from build123d import *

# Parameters (mm, degrees)
BOSS_EXTRUDE1_START = -72.4
SKETCH1_W           = 25.6
SKETCH1_H           = 1.2
BOSS_EXTRUDE1_DEPTH = 16.8
BOSS_EXTRUDE2_START = -71.8
SKETCH2_W           = 24.4
SKETCH2_H           = 1.21
BOSS_EXTRUDE2_DEPTH = 15.6
BOSS_EXTRUDE3_START = -72.1
SKETCH3_W           = 1
SKETCH3_H           = 1.1
BOSS_EXTRUDE3_DEPTH = 0.31
BOSS_EXTRUDE4_START = -56.21
SKETCH4_W           = 1
SKETCH4_H           = 1.1
BOSS_EXTRUDE4_DEPTH = 0.31
BOSS_EXTRUDE5_START = -72.1
SKETCH5_W           = 1
SKETCH5_H           = 1.1
BOSS_EXTRUDE5_DEPTH = 0.31
BOSS_EXTRUDE6_START = -56.21
SKETCH6_W           = 1
SKETCH6_H           = 1.1
BOSS_EXTRUDE6_DEPTH = 0.31
BOSS_EXTRUDE7_START = -72.5
SKETCH7_W           = 3
SKETCH7_H           = 0.7
BOSS_EXTRUDE7_DEPTH = 0.9


with BuildPart() as part:
    # Sketch1 → Boss-Extrude1 (new body)
    with BuildSketch(Plane.XY.offset(BOSS_EXTRUDE1_START)):
        with Locations((-26.8, 0.6)):
            Rectangle(SKETCH1_W, SKETCH1_H)
    extrude(amount=BOSS_EXTRUDE1_DEPTH)

    # Sketch2 → Boss-Extrude2 (add)
    with BuildSketch(Plane.XY.offset(BOSS_EXTRUDE2_START)):
        with Locations((-26.8, 1.795)):
            Rectangle(SKETCH2_W, SKETCH2_H)
    extrude(amount=BOSS_EXTRUDE2_DEPTH)

    # Sketch3 → Boss-Extrude3 (add)
    with BuildSketch(Plane.XY.offset(BOSS_EXTRUDE3_START)):
        with Locations((-21.4, 1.85)):
            Rectangle(SKETCH3_W, SKETCH3_H)
    extrude(amount=BOSS_EXTRUDE3_DEPTH)

    # Sketch4 → Boss-Extrude4 (add)
    with BuildSketch(Plane.XY.offset(BOSS_EXTRUDE4_START)):
        with Locations((-21.4, 1.85)):
            Rectangle(SKETCH4_W, SKETCH4_H)
    extrude(amount=BOSS_EXTRUDE4_DEPTH)

    # Sketch5 → Boss-Extrude5 (add)
    with BuildSketch(Plane.XY.offset(BOSS_EXTRUDE5_START)):
        with Locations((-32.2, 1.85)):
            Rectangle(SKETCH5_W, SKETCH5_H)
    extrude(amount=BOSS_EXTRUDE5_DEPTH)

    # Sketch6 → Boss-Extrude6 (add)
    with BuildSketch(Plane.XY.offset(BOSS_EXTRUDE6_START)):
        with Locations((-32.2, 1.85)):
            Rectangle(SKETCH6_W, SKETCH6_H)
    extrude(amount=BOSS_EXTRUDE6_DEPTH)


with BuildPart() as body_2:
    # Sketch7 → Boss-Extrude7 (new body)
    with BuildSketch(Plane.XY.offset(BOSS_EXTRUDE7_START)):
        with Locations((-26.8, 0.25)):
            Rectangle(SKETCH7_W, SKETCH7_H)
    extrude(amount=BOSS_EXTRUDE7_DEPTH)


with BuildPart() as part_1:
    add(part.part)

    # Combine1: cut body 2
    add(body_2.part, mode=Mode.SUBTRACT)


solid = part_1.part
For this review, take the finished solid that the model builds, in its own axes (mm). A direction names the side the tool comes from. Round coordinates to 2 decimals unless told otherwise and drop trailing zeros. Order: outer loops, then holes, each group sorted by start corner. A loop starts at its lowest first (then second) coordinate and runs counter-clockwise, first axis right, second up. Notation, with made-up numbers: M 51.25,-6 L 76.25,-6 A24 cw 76.25,27 Z; hole C -22,0.25 d5. An arc over 180 degrees is marked long. Use a Markdown table: item, result. Add a question column.
Item 1: Tool access review of faces 1 (the flat face through (-39, 2, -64)), 2 (the flat face through (-27, 0.6, -72)), 3 (the flat face through (-21.4, 1.9, -72.1)): name each direction out of +Z, -Z, +X, -X, +Y, -Y from which nothing blocks a thin tool from reaching the whole face with its end or side.
Item 2: Mouldability with a two-part tool opening along X and no side actions: class faces 4 (the flat face through (-28, 1.2, -56)), 5 (the flat face through (-27, 2, -56.2)), 6 (the flat face through (-14.6, 2, -64)) as released by +X, released by -X, zero draft, split by the parting line, or undercut.
Item 3: To check wall thickness, follow line 1 along X through (y, z) = (1.95, -61.75); line 2 along Z through (x, y) = (-18.5, 1.3). State the ranges of each line that lie inside material, in increasing order.
Item 4: Insertion check: pin 1 (1 mm diameter, centred on y = 2, z = -61.5, fed in from -X); pin 2 (0.5 mm diameter, centred on x = -32.5, y = 2, fed in from -Z). Each pin has a flat end and moves straight along its axis. Give the tip position at first contact, or say it passes through.
Item 5: Add section C-C, the plane x = -23. Give the boundary of the cut face in (y, z), then the cut area to 3 significant figures.
Item 6: Add section A-A, the plane z = -71. Give the boundary of the cut face in (x, y).
Item 7: Add section B-B, the plane y = 1.85. Give the boundary of the cut face in (x, z), then the cut area to 3 significant figures.
Geometry results:
| question | item | result |
|---|---|---|
| 1 | face 1 | +Z, -Z, -X, +Y |
| 1 | face 2 | -Z, -Y |
| 1 | face 3 | -Z, +X, -X, +Y |
| 2 | face 4 | zero draft |
| 2 | face 5 | undercut |
| 2 | face 6 | released by +X |
| 3 | line 1 | x = -39 to -14.6 |
| 3 | line 2 | z = -71.8 to -56.2 |
| 4 | pin 1 | stops at x = -39 |
| 4 | pin 2 | stops at z = -72.1 |
| 5 | outline | M 0,-72.4 L 1.2,-72.4 L 1.2,-71.8 L 2.4,-71.8 L 2.4,-56.2 L 1.2,-56.2 L 1.2,-55.6 L 0,-55.6 Z |
| 5 | area | 38.9 mm² |
| 6 | outline | M -39.6,0 L -14,0 L -14,1.2 L -14.6,1.2 L -14.6,2.4 L -39,2.4 L -39,1.2 L -39.6,1.2 Z |
| 7 | outline | M -39,-71.8 L -32.7,-71.8 L -32.7,-72.1 L -31.7,-72.1 L -31.7,-71.8 L -21.9,-71.8 L -21.9,-72.1 L -20.9,-72.1 L -20.9,-71.8 L -14.6,-71.8 L -14.6,-56.2 L -20.9,-56.2 L -20.9,-55.9 L -21.9,-55.9 L -21.9,-56.2 L -31.7,-56.2 L -31.7,-55.9 L -32.7,-55.9 L -32.7,-56.2 L -39,-56.2 Z |
| 7 | area | 382 mm² |
